The drawing under review shows one solid part. Ordinate dimensions are in mm from its lowest x, y, z. A direction names the side the tool comes from. Give positions to 0.01 mm unless a question says otherwise; leave off trailing zeros. Write each loop counter-clockwise with the first axis right and the second up, starting at its lowest first coordinate (ties: lowest second). Pieces come first, ordered by that corner, then holes. Notation, with made-up numbers: M -14,83.25 L 2,83.25 A18 cw 2,97.25 Z; hole C -26.5,86.5 d7. An arc over 180 degrees is marked long. One line per item, written item: value. Start each with the question number.
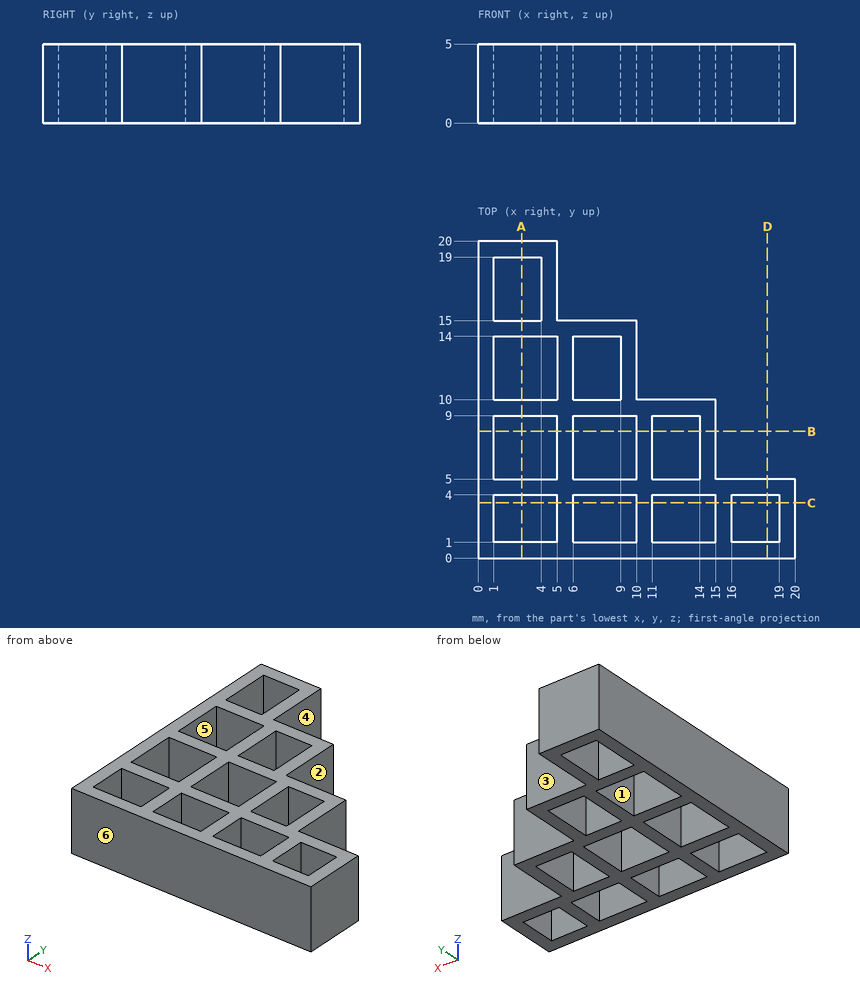
Q1. The part is to be moulded in two halves that separate along Y. For the marked faces 1, 2 and 3, say which applies: pulls with the +Y half, pulls with the -Y half, needs draft (parallel to the pull), parting line crosses it, or undercut.
Q2. Wall thickness on line 1 (X direction, y = 12, z = 4.3); line 2 (Y direction, x = 9.25, z = 0.7); line 3 (Y direction, x = 3, z = 1.55): over which ranges is each line inside the solid? List them lowest first. Write a range as from..to.
Q3. Take a section at B-B, the plane y = 8. Give the boundary of the cut face in (x, z), then the cut area to 3 significant figures.
Q4. For P1, Ø2.5, axis at x = 16.5, z = 1.5, coming from the +Y side; P2, Ø1.5, axis at y = 17.5, z = 2.5, coming from the +X side; P3, Ø3, axis at x = 8.5, z = 2.5, coming from the +Y side; P4, Ø1.5, axis at x = 16.5, y = 6, coming from the -Z side (1 decimal), all flat-tipped, find the tip position at first contact; note any pin that passes through.
Q5. Machinability: for the marked faces 4, 5 and 6, which of the approach directions +Z, -Z, +X, -X, +Y, -Y give a long, thin tool a straight path to every point of the face, cutting with its end or side? Answer none if there is none.
Q6. Take a section at D-D, the plane x = 18.25. Give the boundary of the cut face in (y, z).
Q7. Take a section at C-C, the plane y = 3.5. Give the boundary of the cut face in (x, z), then the cut area to 3 significant figures.
Q8. Take a section at A-A, the plane x = 2.75. Give the boundary of the cut face in (y, z).
Results list:
1. face 1: undercut
1. face 2: needs draft
1. face 3: pulls with the +Y half
2. line 1: x = 0..1, 5..6, 9..10
2. line 2: y = 0..1, 4..5, 9..15
2. line 3: y = 0..1, 4..5, 9..10, 14..15, 19..20
3. outline: M 0,0 L 1,0 L 1,5 L 0,5 Z; M 5,0 L 6,0 L 6,5 L 5,5 Z; M 10,0 L 11,0 L 11,5 L 10,5 Z; M 14,0 L 15,0 L 15,5 L 14,5 Z
3. area: 20.0 mm^2
4. P1: stops at y = 5
4. P2: stops at x = 5
4. P3: stops at y = 15
4. P4: passes through
5. face 4: +Z, -Z, +X, +Y
5. face 5: +Z, -Z
5. face 6: +Z, -Z, +X, -X, -Y
6. outline: M 0,0 L 1,0 L 1,5 L 0,5 Z; M 4,0 L 5,0 L 5,5 L 4,5 Z
7. outline: M 0,0 L 1,0 L 1,5 L 0,5 Z; M 5,0 L 6,0 L 6,5 L 5,5 Z; M 10,0 L 11,0 L 11,5 L 10,5 Z; M 15,0 L 16,0 L 16,5 L 15,5 Z; M 19,0 L 20,0 L 20,5 L 19,5 Z
7. area: 25.0 mm^2
8. outline: M 0,0 L 1,0 L 1,5 L 0,5 Z; M 4,0 L 5,0 L 5,5 L 4,5 Z; M 9,0 L 10,0 L 10,5 L 9,5 Z; M 14,0 L 15,0 L 15,5 L 14,5 Z; M 19,0 L 20,0 L 20,5 L 19,5 Z
